Can you work these out from the model? Positions are in its coordinate system, mm. A direction names the side the tool comes from. Give positions to 0.01 mm unless a question says otherwise; leave off trailing zeros. Order: outer loops, then holes, each group sorted by start corner. A loop starts at its lowest first (then second) coordinate and runs counter-clockwise, first axis right, second up. Notation, with made-up numbers: (63.25, -34.75) -> (70.25, -34.75) arc R27 cw to (70.25, -14.75) -> close; hole circle Ø4 at (41.5, 22.5). An arc over 180 degrees is marked (long way). Answer as a JSON object with one key per item and string values.
```python
from build123d import *

# Parameters (mm, degrees)
F0_R     = 365.125
F1_DEPTH = 19.05
F2_R     = 120.65
F2_R_2   = 101.6
F3_DEPTH = 304.8
F4_R     = 365.125
F4_R_2   = 120.65
F4_R_3   = 101.6
F5_DEPTH = 19.05
F6_R     = 38.1
F7_DEPTH = 355.6
F8_R     = 12.7
F9_DEPTH = 355.6


with BuildPart() as f1:
    # F0 (on Top) → F1 (new body)
    with BuildSketch(Plane.XY):
        Circle(F0_R)
    extrude(amount=F1_DEPTH)

    # F2 (on face) → F3 (join)
    with BuildSketch(Plane.XY.offset(19.05)):
        Circle(F2_R)
        Circle(F2_R_2, mode=Mode.SUBTRACT)
    extrude(amount=F3_DEPTH)

    # F4 (on face) → F5 (join)
    with BuildSketch(Plane.XY.offset(323.85)):
        Circle(F4_R)
        Circle(F4_R_2, mode=Mode.SUBTRACT)
        Circle(F4_R_2)
        Circle(F4_R_3, mode=Mode.SUBTRACT)
        Circle(F4_R_3)
    extrude(amount=F5_DEPTH)

    # F6 (on face) → F7 (cut)
    with BuildSketch(Plane(origin=(0, 0, 0), x_dir=(1, 0, 0), z_dir=(0, 0, -1))):
        Circle(F6_R)
    extrude(amount=-F7_DEPTH, mode=Mode.SUBTRACT)

    # F8 (on face) → F9 (cut)
    with BuildSketch(Plane.XY.offset(342.9)):
        with Locations((-81.28, 0)):
            Circle(F8_R)
        with Locations((81.28, 0)):
            Circle(F8_R)
    extrude(amount=-F9_DEPTH, mode=Mode.SUBTRACT)


solid = f1.part
```
1. For faces 5 (the face through (-5, -76, 342.9)), 6 (the face through (44, 1, 19.05)), which set-ups out of +Z, -Z, +X, -X, +Y, -Y let a thin tool reach every point of the face, with its end or its side?
Worked answers:
{"face 5": "+Z, +X, -X, +Y, -Y", "face 6": "none"}
2. Will these pins go through, and if not, where does the flat tip stop? pin 1 Ø1 at (y, z) = (-34, 239) entering from +X; pin 2 Ø6 at (y, z) = (75.5, 244.5) entering from -X; pin 3 Ø4 at (y, z) = (79, 219) entering from +X.
Worked answers:
{"pin 1": "x = 115.91", "pin 2": "x = -96.44", "pin 3": "x = 92.88"}
3. If we section it at A-A on x = 0: Please give me the cut outline in (y, z) (3 decimals).
Worked answers:
{"outline": "(-365.125, 0) -> (-38.1, 0) -> (-38.1, 19.05) -> (-101.6, 19.05) -> (-101.6, 323.85) -> (-38.1, 323.85) -> (-38.1, 342.9) -> (-365.125, 342.9) -> (-365.125, 323.85) -> (-120.65, 323.85) -> (-120.65, 19.05) -> (-365.125, 19.05) -> close; (38.1, 0) -> (365.125, 0) -> (365.125, 19.05) -> (120.65, 19.05) -> (120.65, 323.85) -> (365.125, 323.85) -> (365.125, 342.9) -> (38.1, 342.9) -> (38.1, 323.85) -> (101.6, 323.85) -> (101.6, 19.05) -> (38.1, 19.05) -> close"}
4. If we mould it in two halves opening along Y, with no side actions, what happens to faces 1 (the face through (-86, 86, 323.85)), 2 (the face through (68.592, 0.558, 9.658)), 3 (the face through (348.264, 109.674, 9.392)), 4 (the face through (-30.235, 23.183, 9.392))? For each: +Y half, -Y half, draft (parallel to the pull), parting line (faces both ways), or undercut.
Worked answers:
{"face 1": "draft", "face 2": "undercut", "face 3": "parting line", "face 4": "undercut"}
5. If we section it at C-C on z = 29.5: Please give me the cut outline in (x, y).
Worked answers:
{"outline": "circle Ø241.3 at (0, 0); hole circle Ø203.2 at (0, 0)"}
6. Please list where these lines run through material, in increasing order: L1, parallel to Z at x = -265, y = 49.5; L2, parallel to Y at x = 0, z = 14 (3 decimals); L3, parallel to X at y = 78, z = 137.5.
Worked answers:
{"L1": "0 to 19.05, 323.85 to 342.9", "L2": "-365.125 to -38.1, 38.1 to 365.125", "L3": "-92.05 to -65.1, 65.1 to 92.05"}
7. If we section it at B-B on y = 209.5: Please give me the cut outline in (x, z), then the cut area to 3 significant figures.
Worked answers:
{"outline": "(-299.04, 0) -> (299.04, 0) -> (299.04, 19.05) -> (-299.04, 19.05) -> close; (-299.04, 323.85) -> (299.04, 323.85) -> (299.04, 342.9) -> (-299.04, 342.9) -> close", "area": "22,800 mm²"}
8. If we section it at D-D on y = 0: Count the separate pieces of the cut face and the enclosed holes in it, then the cut area to 3 significant figures.
Worked answers:
{"separate pieces": "6", "enclosed holes": "0", "area": "34,600 mm²"}
